Part model, mm, in its own coordinate system. A direction names the side the tool comes from. Give positions to 0.01 mm unless a question says otherwise; leave off trailing zeros. Write each loop counter-clockwise with the first axis right and the second up, starting at its lowest first coordinate (ties: lowest second). Pieces come first, ordered by that corner, then holes.
from build123d import *

# Parameters (mm, degrees)
SKETCH1_W           = 63
SKETCH1_H           = 70
BOSS_EXTRUDE1_DEPTH = 21
SKETCH2_W           = 10
SKETCH2_H           = 21
BOSS_EXTRUDE2_DEPTH = 5
FILLET3_R           = 3
FILLET4_R           = 1.5


with BuildPart() as part:
    # Sketch1 → Boss-Extrude1 (new body)
    with BuildSketch(Plane(origin=(0, 0, 0), x_dir=(1, 0, 0), z_dir=(0, 1, 0))):
        Rectangle(SKETCH1_W, SKETCH1_H)
    extrude(amount=BOSS_EXTRUDE1_DEPTH)

    # Sketch2 → Boss-Extrude2 (add)
    with BuildSketch(Plane(origin=(31.5, 0, 0), x_dir=(0, 0, -1), z_dir=(1, 0, 0))):
        with Locations((30, 10.5)):
            Rectangle(SKETCH2_W, SKETCH2_H)
    extrude(amount=BOSS_EXTRUDE2_DEPTH)

    # Fillet3
    fillet3_edges = [part.edges().sort_by_distance(p)[0] for p in [
        (31.5, 0, 5),
        (31.5, 21, 5),
        (36.5, 21, -30),
        (36.5, 0, -30),
        (-31.5, 21, 0),
        (-31.5, 0, 0),
    ]]
    fillet(fillet3_edges, radius=FILLET3_R)

    # Fillet4
    fillet4_edges = [part.edges().sort_by_distance(p)[0] for p in [
        (-31.5, 10.5, 35),
        (-31.5, 10.5, -35),
        (0, 0, 35),
        (31.5, 10.5, 35),
        (0, 21, 35),
        (30.621320344, 20.121320344, 35),
        (30.621320344, 0.878679656, 35),
        (-30.621320344, 20.121320344, 35),
        (-30.621320344, 0.878679656, 35),
        (2.5, 0, -35),
        (2.5, 21, -35),
        (36.5, 10.5, -35),
        (35.621320344, 20.121320344, -35),
        (35.621320344, 0.878679656, -35),
        (-30.621320344, 20.121320344, -35),
        (-30.621320344, 0.878679656, -35),
    ]]
    fillet(fillet4_edges, radius=FILLET4_R)


solid = part.part
1) 3-axis set-ups, long thin cutter, end or side, ignore diameter. For faces 1 (the flat face through (31.5, 10, 5)), 2 (the cylindrical face through (0.4, 20.55, 34.57)), 3 (the cylindrical face through (30.64, 0.9, 3.84)): which of +Z, -Z, +X, -X, +Y, -Y reach the whole face in a straight line?
Check result:
face 1: +Z, +X, +Y, -Y
face 2: +Z, +X, -X, +Y
face 3: +Z, +X, -Y
2) Saw through at A-A (y = 16.25). Write the cut outline in (x, z).
Check result:
outline: (-31.5, -33.5) arc R1.5 ccw to (-30, -35) - (35, -35) arc R1.5 ccw to (36.5, -33.5) - (36.5, -25) - (31.5, -25) - (31.5, 33.5) arc R1.5 ccw to (30, 35) - (-30, 35) arc R1.5 ccw to (-31.5, 33.5) - close
3) Flat gauge pin, fed straight in: P1, Ø2, axis at y = 18, z = -14.5, coming from the +X side. Where does the tip first touch, or does it go through?
Check result:
P1: stops at x = 31.5
4) Drill centre lines: L1, parallel to X at y = 12, z = -18.5; L2, parallel to Z at x = 31, y = 3.25. Where is each one in solid material? Low to high.
Check result:
L1: x = -31.5 to 31.5
L2: z = -35 to 34.62
5) Saw through at B-B (z = 25). Write the cut outline in (x, y).
Check result:
outline: (-31.5, 3) arc R3 ccw to (-28.5, 0) - (28.5, 0) arc R3 ccw to (31.5, 3) - (31.5, 18) arc R3 ccw to (28.5, 21) - (-28.5, 21) arc R3 ccw to (-31.5, 18) - close
